Input: part model. Units: mm. Frame: model coordinates. A direction names the side the tool comes from. Round coordinates to 2 decimals unless told otherwise and drop trailing zeros. Loops run counter-clockwise (first coordinate to the right, second up) from the corner with the lowest first, then second, coordinate; pieces in that order, holes last.
(1) Cut plane A-A, the plane x = 9.5. Output: boundary loops of the cut face in (y, z).
(2) First-contact query: pin 1 Ø8 at (x, y) = (3.5, -1) entering from +Z; pin 2 Ø6 at (x, y) = (16, -5.5) entering from -Z; pin 3 Ø6 at (y, z) = (-1.5, 7) entering from +X; pin 4 Ø3 at (x, y) = (3.5, 2) entering from +Z. Flat tips, straight axial feed; report the tip coordinate or a pass-through.
(3) Access query for faces 1 (the face through (0, 7, -3)), 2 (the face through (-5, 0, -12)), 3 (the face through (-0.39, -2.38, -10.74)). Directions: +Z, -Z, +X, -X, +Y, -Y. A direction counts if a zero-diameter tool reaches every point of the face in a straight line with its end or side. Return the directions, or none.
(4) Line query: line 1 (X direction, y = 7.25, z = 8.75); line 2 (X direction, y = 3.75, z = 6.5); line 3 (X direction, y = -8, z = 6). Output: solid intervals per line, ascending.
Autodesk Inventor part; units mm, degrees
ref_plane "YZ Plane" through (0, 0, 0) normal (1, 0, 0) x (0, 1, 0)
ref_plane "XZ Plane" through (0, 0, 0) normal (0, 1, 0) x (-1, 0, 0)
ref_plane "XY Plane" through (0, 0, 0) normal (0, 0, 1) x (1, 0, 0)
sketch "Skizze1" plane through (0, 0, 0) normal (0, 0, 1) x (1, 0, 0)
  line L0 (0, 11) -> (0, 7.4587)
  line L1 (6, 8) -> (40, 8)
  line L2 (40, 8) -> (40, 0)
  line L3 (40, 0) -> (-0.8001, 0)
  line L4 (-4.8801, 0) -> (52.24, 0)
  line L5 (-0.8001, 0) -> (-0.8001, 11)
  line L6 (-0.8001, 11) -> (0, 11)
  line L7 (6, 8) -> (4.773, 7.4587)
  line L8 (4.773, 7.4587) -> (0, 7.4587)
  line L9 (0, -1.1) -> (0, 14.3)
  dimension "d0" = 40
  dimension "d1" = 34
  dimension "d2" = 16
  dimension "d9" = 0.8001
  dimension "d10" = 22
  dimension "d13" = 1.227
  dimension "d14" = 14.9175
revolve "Körper" add sketch "Skizze1" angle 360 about axis through (40, 0, 0) along (-1, 0, 0)
sketch "Skizze2" plane through (-0.8001, 0, 0) normal (-1, 0, 0) x (0, 0, 1)
  line L0 (0, 13.8564) -> (12, 6.9282)
  line L1 (12, 6.9282) -> (12, -6.9282)
  line L2 (12, -6.9282) -> (0, -13.8564)
  line L3 (0, -13.8564) -> (-12, -6.9282)
  line L4 (-12, -6.9282) -> (-12, 6.9282)
  line L5 (-12, 6.9282) -> (0, 13.8564)
  point P0 (0, 0)
  point P1 (0, 0)
  dimension "d11" = 24
extrude "Kopf" add sketch "Skizze2" along normal blind 9.2
sketch "Skizze4" plane through (0, 0, 0) normal (0, 0, 1) x (1, 0, 0)
  line L0 (-10.0001, 12) -> (-10.0001, 13.8564)
  line L1 (-10.0001, 13.8564) -> (-8.9283, 13.8564)
  line L2 (-8.9283, 13.8564) -> (-10.0001, 12)
  line L3 (-10.9201, 0) -> (1.9599, 0)
  line L4 (-0.8001, 13.8564) -> (-10.0001, 13.8564)
  line L5 (-10.0001, 6.9282) -> (-10.0001, 13.8564)
  dimension "d5" = 30
  dimension "d19" = 24
revolve "Fase1" cut sketch "Skizze4" angle 360 about axis through (-10, 0, 0) along (1, 0, 0)
thread "Gewinde"
chamfer "Fase2" distance 1.2269 distance2 1.227 1 edges at (40, -8, 0) measured on face at (40, -0.1598, 1.3157)
equation "\"d0\" = NLG"
equation "\"d1\" = GEL"
equation "\"d2\" = GD"
equation "\"d10\" = SD2"
equation "\"d14\" = BDM"
equation "\"d11\" = SW"
equation "\"d3\" = KOH - SD"
equation "\"d5\" = ANG1"
equation "\"d19\" = SW0"
equation "\"d15\" = GEL"
equation "\"d6\" = -0.5 * SPD + 0.5 * GD"
equation "\"NLG\" = 40"
equation "\"GD\" = NND"
equation "\"BDM\" = 14.91747"
equation "\"KOH\" = 10"
equation "\"GEL\" = 34"
equation "\"SW\" = 24"
equation "\"SW0\" = 24"
equation "\"SPD\" = NND - 1.2269 * TPU"
equation "\"SD2\" = 22"
equation "\"SD\" = 0.8"
equation "\"ANG1\" = 30deg"
equation "\"GAL\" = 0.61345 * TPU"
equation "\"GUL\" = 0.61345 * TPU"
equation "\"RR\" = 0.6"
equation "\"TOA\" = 30deg"
equation "\"PTC\" = TPU"
equation "\"GD1\" = THREADDIA - 1.2269 * TPU"
equation "\"TPU\" = 2"
equation "\"THREADDIA\" = 16"
equation "\"E0\" = 1.155 * SW"
equation "\"NND\" = 16"
properties part number "DIN 933 - M16  x 40"
Reported:
1. outline: circle Ø16 at (0, 0)
2. pin 1: stops at z = 11
2. pin 2: stops at z = -7.6
2. pin 3: stops at x = 40
2. pin 4: stops at z = 7.44
3. face 1: none
3. face 2: -Z, +X, -X, +Y, -Y
3. face 3: +X
4. line 1: x = -10 to -0.8
4. line 2: x = -10 to 0, 4.88 to 39.27
4. line 3: x = -10 to 0
